```python
from build123d import *

# Parameters (mm, degrees)
SKETCH_2_W          = 330
SKETCH_2_H          = 110
SKETCH_2_R          = 2
EXTRUDE_1_DEPTH     = 3
CUT_EXTRUDE_1_DEPTH = 198.929546993
FILLET_1_R          = 20


with BuildPart() as part:
    # 草图2 → 凸台-拉伸1 (new body)
    with BuildSketch(Plane.XY):
        with Locations((20.115321252, 14.995881384)):
            Rectangle(SKETCH_2_W, SKETCH_2_H)
        with Locations((-109.884678748, 59.995881384)):
            Circle(SKETCH_2_R, mode=Mode.SUBTRACT)
        with Locations(Location((150.115321252, 59.995881384, 0), (0, 0, 180))):
            Circle(SKETCH_2_R, mode=Mode.SUBTRACT)
        with Locations((-69.884678748, -30.004118616)):
            Circle(SKETCH_2_R, mode=Mode.SUBTRACT)
        with Locations(Location((110.115321252, -30.004118616, 0), (0, 0, 180))):
            Circle(SKETCH_2_R, mode=Mode.SUBTRACT)
    extrude(amount=EXTRUDE_1_DEPTH)

    # 草图3 → 切除-拉伸1 (cut, through all)
    with BuildSketch(Plane.XY.offset(3)):
        with BuildLine():
            Line((16.115321252, -7.504118616), (16.115321252, 37.495881384))
            ThreePointArc((16.115321252, 37.495881384), (20.115321252, 41.495881384), (24.115321252, 37.495881384))
            Line((24.115321252, 37.495881384), (24.115321252, -7.504118616))
            ThreePointArc((24.115321252, -7.504118616), (20.115321252, -11.504118616), (16.115321252, -7.504118616))
        make_face()
        with BuildLine():
            Line((41.115321252, -7.504118616), (41.115321252, 37.495881384))
            ThreePointArc((41.115321252, 37.495881384), (45.115321252, 41.495881384), (49.115321252, 37.495881384))
            Line((49.115321252, 37.495881384), (49.115321252, -7.504118616))
            ThreePointArc((49.115321252, -7.504118616), (45.115321252, -11.504118616), (41.115321252, -7.504118616))
        make_face()
        with BuildLine():
            Line((66.115321252, -7.504118616), (66.115321252, 37.495881384))
            ThreePointArc((66.115321252, 37.495881384), (70.115321252, 41.495881384), (74.115321252, 37.495881384))
            Line((74.115321252, 37.495881384), (74.115321252, -7.504118616))
            ThreePointArc((74.115321252, -7.504118616), (70.115321252, -11.504118616), (66.115321252, -7.504118616))
        make_face()
        with BuildLine():
            Line((91.115321252, -7.504118616), (91.115321252, 37.495881384))
            ThreePointArc((91.115321252, 37.495881384), (95.115321252, 41.495881384), (99.115321252, 37.495881384))
            Line((99.115321252, 37.495881384), (99.115321252, -7.504118616))
            ThreePointArc((99.115321252, -7.504118616), (95.115321252, -11.504118616), (91.115321252, -7.504118616))
        make_face()
        with BuildLine():
            Line((116.115321252, -7.504118616), (116.115321252, 37.495881384))
            ThreePointArc((116.115321252, 37.495881384), (120.115321252, 41.495881384), (124.115321252, 37.495881384))
            Line((124.115321252, 37.495881384), (124.115321252, -7.504118616))
            ThreePointArc((124.115321252, -7.504118616), (120.115321252, -11.504118616), (116.115321252, -7.504118616))
        make_face()
        with BuildLine():
            Line((141.115321252, -7.504118616), (141.115321252, 37.495881384))
            ThreePointArc((141.115321252, 37.495881384), (145.115321252, 41.495881384), (149.115321252, 37.495881384))
            Line((149.115321252, 37.495881384), (149.115321252, -7.504118616))
            ThreePointArc((149.115321252, -7.504118616), (145.115321252, -11.504118616), (141.115321252, -7.504118616))
        make_face()
        with BuildLine():
            Line((-0.884678748, -7.504118616), (-0.884678748, 37.495881384))
            ThreePointArc((-0.884678748, 37.495881384), (-4.884678748, 41.495881384), (-8.884678748, 37.495881384))
            Line((-8.884678748, 37.495881384), (-8.884678748, -7.504118616))
            ThreePointArc((-8.884678748, -7.504118616), (-4.884678748, -11.504118616), (-0.884678748, -7.504118616))
        make_face()
        with BuildLine():
            Line((-25.884678748, -7.504118616), (-25.884678748, 37.495881384))
            ThreePointArc((-25.884678748, 37.495881384), (-29.884678748, 41.495881384), (-33.884678748, 37.495881384))
            Line((-33.884678748, 37.495881384), (-33.884678748, -7.504118616))
            ThreePointArc((-33.884678748, -7.504118616), (-29.884678748, -11.504118616), (-25.884678748, -7.504118616))
        make_face()
        with BuildLine():
            Line((-50.884678748, -7.504118616), (-50.884678748, 37.495881384))
            ThreePointArc((-50.884678748, 37.495881384), (-54.884678748, 41.495881384), (-58.884678748, 37.495881384))
            Line((-58.884678748, 37.495881384), (-58.884678748, -7.504118616))
            ThreePointArc((-58.884678748, -7.504118616), (-54.884678748, -11.504118616), (-50.884678748, -7.504118616))
        make_face()
        with BuildLine():
            Line((-75.884678748, -7.504118616), (-75.884678748, 37.495881384))
            ThreePointArc((-75.884678748, 37.495881384), (-79.884678748, 41.495881384), (-83.884678748, 37.495881384))
            Line((-83.884678748, 37.495881384), (-83.884678748, -7.504118616))
            ThreePointArc((-83.884678748, -7.504118616), (-79.884678748, -11.504118616), (-75.884678748, -7.504118616))
        make_face()
        with BuildLine():
            Line((-100.884678748, -7.504118616), (-100.884678748, 37.495881384))
            ThreePointArc((-100.884678748, 37.495881384), (-104.884678748, 41.495881384), (-108.884678748, 37.495881384))
            Line((-108.884678748, 37.495881384), (-108.884678748, -7.504118616))
            ThreePointArc((-108.884678748, -7.504118616), (-104.884678748, -11.504118616), (-100.884678748, -7.504118616))
        make_face()
    extrude(amount=-CUT_EXTRUDE_1_DEPTH, mode=Mode.SUBTRACT)

    # 圆角1
    fillet_1_edges = [part.edges().sort_by_distance(p)[0] for p in [
        (-144.884678748, 69.995881384, 1.5),
        (185.115321252, 69.995881384, 1.5),
        (185.115321252, -40.004118616, 1.5),
        (-144.884678748, -40.004118616, 1.5),
    ]]
    fillet(fillet_1_edges, radius=FILLET_1_R)


solid = part.part
```
Part model, mm, in its own coordinate system. Coordinates: 2 decimals unless noted, no trailing zeros. Return JSON: item names as keys, results as strings. Group by question number.
Item 1: Cut at A-A (y = 4). State how many separate pieces and enclosed holes the cut face has, plus the area to 3 significant figures.
Item 2: Pin check, flat tip, straight feed: pin 1 (3 mm diameter, centred on x = -54, y = 27.5, fed in from +Z). Stop position of the tip, or through.
Item 3: Drill centre lines: probe 1 along Y at (x, z) = (70, 0.6); probe 2 along X at (y, z) = (-29, 0.1); probe 3 along Y at (x, z) = (-105.5, 1.3). Where is each one in solid material? Low to high. Write a range as from..to.
Check values:
{
 "1": {"separate pieces": "12", "enclosed holes": "0", "area": "726 mm2"},
 "2": {"pin 1": "passes through"},
 "3": {"probe 1": "y = -40..-11.5, 41.49..70", "probe 2": "x = -142.75..-71.61, -68.16..108.39, 111.84..182.98", "probe 3": "y = -40..-11.46, 41.45..70"}
}
